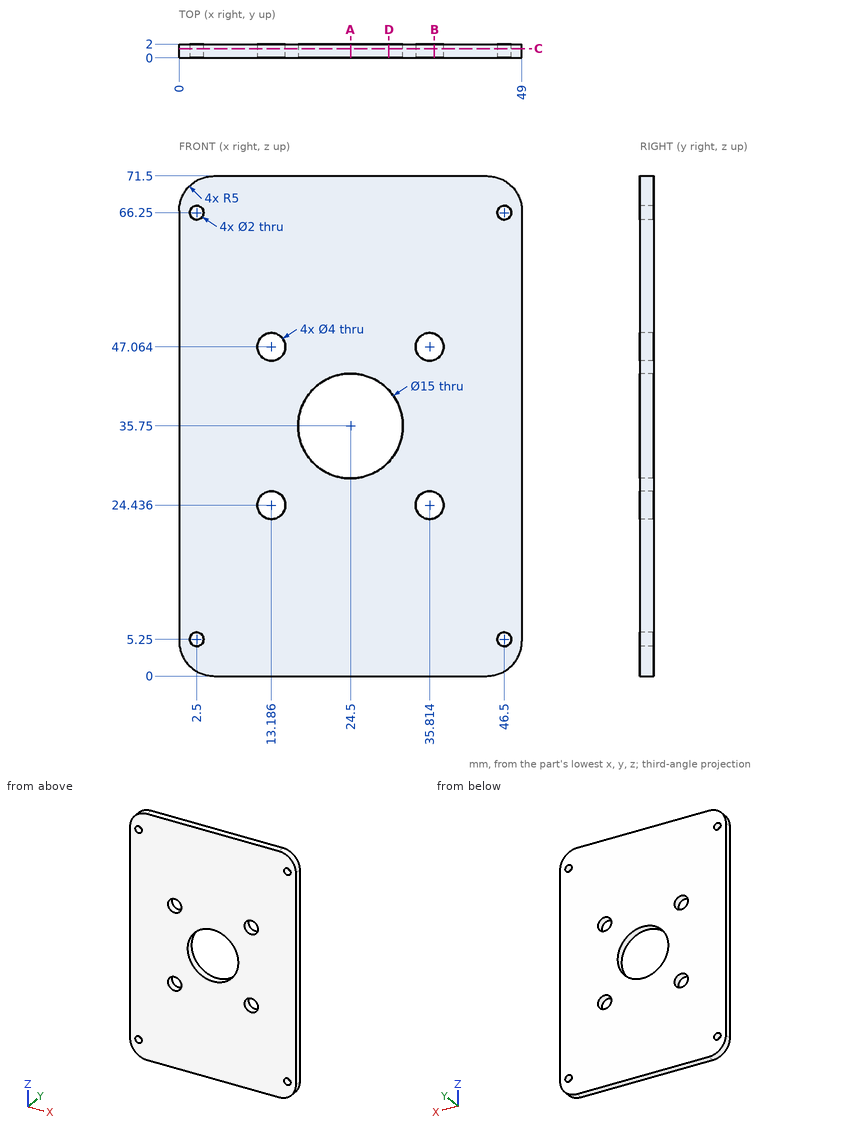
For this review, use the dimensioned drawing (mm, ordinates from the lowest corner) and the shaded views. Round coordinates to 2 decimals unless told otherwise and drop trailing zeros. Order: outer loops, then holes, each group sorted by start corner. A loop starts at its lowest first (then second) coordinate and runs counter-clockwise, first axis right, second up. Notation, with made-up numbers: (-8, -1) -> (35, -1) arc R27 ccw to (35, 37) -> close; hole circle Ø11 at (-37, -4.75). An arc over 180 degrees is marked (long way). Write item = value, one per line. Start each with the question number.
Item 1: Clearance check with a flat-ended pin moving along its axis: pin 1 Ø2 at (x, z) = (26.5, 41.5) entering from +Y. State where the tip first meets the part, or that it passes through.
Item 2: For line 1 along X through (y, z) = (0.65, 35.75); line 2 along X through (y, z) = (1.55, 66.25); line 3 along Z through (x, y) = (36.5, 1.6) (1 decimal), list the stretches that pass through material, from the lowest coordinate up.
Item 3: Consider section D-D on x = 30. Write out the cut boundary in (y, z), plus the area to 3 significant figures.
Item 4: Consider section B-B on x = 36.5. Write out the cut boundary in (y, z) (1 decimal), plus the area to 3 significant figures.
Item 5: Consider section C-C on y = 1.35. Count the separate pieces of the cut face and the enclosed holes in it, plus the area to 3 significant figures.
Item 6: Consider section A-A on x = 24.5. Write out the cut boundary in (y, z), plus the area to 3 significant figures.
Conclusion:
q1.pin_1 = through
q2.line_1 = 0 to 17, 32 to 49
q2.line_2 = 0 to 1.5, 3.5 to 45.5, 47.5 to 49
q2.line_3 = 0 to 22.6, 26.3 to 45.2, 48.9 to 71.5
q3.outline = (0, 0) -> (2, 0) -> (2, 30.65) -> (0, 30.65) -> close; (0, 40.85) -> (2, 40.85) -> (2, 71.5) -> (0, 71.5) -> close
q3.area = 123 mm2
q4.outline = (0, 0) -> (2, 0) -> (2, 22.6) -> (0, 22.6) -> close; (0, 26.3) -> (2, 26.3) -> (2, 45.2) -> (0, 45.2) -> close; (0, 48.9) -> (2, 48.9) -> (2, 71.5) -> (0, 71.5) -> close
q4.area = 128 mm2
q5.separate_pieces = 1
q5.enclosed_holes = 9
q5.area = 3,240 mm2
q6.outline = (0, 0) -> (2, 0) -> (2, 28.25) -> (0, 28.25) -> close; (0, 43.25) -> (2, 43.25) -> (2, 71.5) -> (0, 71.5) -> close
q6.area = 113 mm2
